Read the model definition and answer for the solid it produces. Units are mm, in the model's axes. A direction names the side the tool comes from. Give positions to 0.01 mm unless a question says otherwise; leave off trailing zeros. Order: outer loops, then holes, each group sorted by start corner. A loop starts at its lowest first (then second) coordinate and runs counter-clockwise, first axis right, second up.
Item 1: The mould has two halves that part along Y. Classify faces 3 (the face through (75, 0, 4)), 4 (the face through (74, 37, 7.873)), 5 (the face through (39.423, 57.426, 6.394)): +Y half, -Y half, draft (parallel to the pull), parting line (faces both ways), or undercut.
Item 2: Which of the six approach directions +Z, -Z, +X, -X, +Y, -Y give full straight-line access (tool end or side, diameter ignored) to faces 1 (the face through (40, 5, 2)), 2 (the face through (136.047, 35.734, 6.394))?
Item 3: A cutting plane is placed at A-A (x = 140). Write down the section's boundary in (y, z).
Item 4: Given pin 1 Ø3 at (x, y) = (15.8, 36.5) entering from -Z; pin 2 Ø3 at (x, y) = (62.5, 35) entering from -Z, each flat-ended and moving along its own axis, determine where each tip first touches the part or whether it passes through.
Item 5: Find the intervals of material crossed by line 1 along X through (y, z) = (11, 1.5); line 2 along Y through (x, z) = (51.25, 5.5); line 3 along X through (y, z) = (13.8, 6.8), in increasing order.
from build123d import *

# Parameters (mm, degrees)
F0_W      = 150
F0_H      = 73
F1_DEPTH  = 7.873
F2_W      = 136
F2_H      = 63
F3_DEPTH  = 4.873
F4_R      = 1.25
F5_DEPTH  = 7.873
F6_R      = 1.25
F7_DEPTH  = 7.873
F8_R      = 1.25
F9_DEPTH  = 7.873
F10_R     = 1.25
F11_DEPTH = 7.873
F12_R     = 1.25
F13_DEPTH = 7.873
F14_R     = 1.25
F15_DEPTH = 7.873
F16_R     = 1.25
F17_DEPTH = 7.873
F18_R     = 1.25
F19_DEPTH = 7.873
F20_R     = 1.25
F21_DEPTH = 7.873
F22_R     = 1.25
F23_DEPTH = 7.873
F24_R     = 1.25
F25_DEPTH = 7.873
F26_R     = 1.25
F27_DEPTH = 7.873
F28_R     = 1.25
F29_DEPTH = 7.873
F30_R     = 1.25
F31_DEPTH = 7.873
F32_R     = 1.25
F33_DEPTH = 7.873
F34_R     = 1.25
F35_DEPTH = 7.873
F36_R     = 1.25
F37_DEPTH = 7.873
F38_R     = 1.25
F39_DEPTH = 7.873
F40_R     = 1.25
F41_DEPTH = 7.873
F42_R     = 1.25
F43_DEPTH = 7.873
F44_R     = 1.25
F45_DEPTH = 7.873
F46_R     = 2
F47_DEPTH = 3
F48_R     = 2
F49_DEPTH = 3
F50_R     = 2
F51_DEPTH = 3
F52_R     = 2
F53_DEPTH = 3
F54_R     = 2
F55_DEPTH = 3
F56_R     = 2
F57_DEPTH = 3
F58_R     = 2
F59_DEPTH = 3
F60_R     = 2
F61_DEPTH = 3
F62_R     = 2
F63_DEPTH = 3
F64_R     = 2
F65_DEPTH = 3
F66_W     = 2.5
F66_H     = 4.873
F67_DEPTH = 63
F68_W     = 2.5
F68_H     = 6.5
F69_DEPTH = 0.623
F70_R     = 2
F71_DEPTH = 3
F73_R     = 2
F74_DEPTH = 3
F75_R     = 2
F76_DEPTH = 3
F77_R     = 2
F78_DEPTH = 3
F79_R     = 2
F80_DEPTH = 3
F72_R     = 2
F81_DEPTH = 3
F82_R     = 1.25
F83_DEPTH = 7.873
F84_R     = 1.25
F85_DEPTH = 7.873


with BuildPart() as f1:
    # F0 (on Top) → F1 (new body)
    with BuildSketch(Plane.XY):
        with Locations((75, 36.5)):
            Rectangle(F0_W, F0_H)
    extrude(amount=F1_DEPTH)

    # F2 (on Top) → F3 (cut)
    with BuildSketch(Plane.XY):
        with Locations((75, 36.5)):
            Rectangle(F2_W, F2_H)
    extrude(amount=F3_DEPTH, mode=Mode.SUBTRACT)

    # F4 (on face) → F5 (cut)
    with BuildSketch(Plane.XY.offset(7.873)):
        with Locations((2.5, 2.5)):
            Circle(F4_R)
    extrude(amount=-F5_DEPTH, mode=Mode.SUBTRACT)

    # F6 (on face) → F7 (cut)
    with BuildSketch(Plane.XY.offset(7.873)):
        with Locations((18, 2.5)):
            Circle(F6_R)
    extrude(amount=-F7_DEPTH, mode=Mode.SUBTRACT)

    # F8 (on face) → F9 (cut)
    with BuildSketch(Plane.XY.offset(7.873)):
        with Locations((34.5, 2.5)):
            Circle(F8_R)
    extrude(amount=-F9_DEPTH, mode=Mode.SUBTRACT)

    # F10 (on face) → F11 (cut)
    with BuildSketch(Plane.XY.offset(7.873)):
        with Locations((51, 2.5)):
            Circle(F10_R)
    extrude(amount=-F11_DEPTH, mode=Mode.SUBTRACT)

    # F12 (on face) → F13 (cut)
    with BuildSketch(Plane.XY.offset(7.873)):
        with Locations((67.5, 2.5)):
            Circle(F12_R)
    extrude(amount=-F13_DEPTH, mode=Mode.SUBTRACT)

    # F14 (on face) → F15 (cut)
    with BuildSketch(Plane.XY.offset(7.873)):
        with Locations((82.5, 2.5)):
            Circle(F14_R)
    extrude(amount=-F15_DEPTH, mode=Mode.SUBTRACT)

    # F16 (on face) → F17 (cut)
    with BuildSketch(Plane.XY.offset(7.873)):
        with Locations((99, 2.5)):
            Circle(F16_R)
    extrude(amount=-F17_DEPTH, mode=Mode.SUBTRACT)

    # F18 (on face) → F19 (cut)
    with BuildSketch(Plane.XY.offset(7.873)):
        with Locations((115.5, 2.5)):
            Circle(F18_R)
    extrude(amount=-F19_DEPTH, mode=Mode.SUBTRACT)

    # F20 (on face) → F21 (cut)
    with BuildSketch(Plane.XY.offset(7.873)):
        with Locations((132, 2.5)):
            Circle(F20_R)
    extrude(amount=-F21_DEPTH, mode=Mode.SUBTRACT)

    # F22 (on face) → F23 (cut)
    with BuildSketch(Plane.XY.offset(7.873)):
        with Locations((147.5, 2.5)):
            Circle(F22_R)
    extrude(amount=-F23_DEPTH, mode=Mode.SUBTRACT)

    # F24 (on face) → F25 (cut)
    with BuildSketch(Plane.XY.offset(7.873)):
        with Locations((2.5, 22)):
            Circle(F24_R)
    extrude(amount=-F25_DEPTH, mode=Mode.SUBTRACT)

    # F26 (on face) → F27 (cut)
    with BuildSketch(Plane.XY.offset(7.873)):
        with Locations((147.5, 22)):
            Circle(F26_R)
    extrude(amount=-F27_DEPTH, mode=Mode.SUBTRACT)

    # F28 (on face) → F29 (cut)
    with BuildSketch(Plane.XY.offset(7.873)):
        with Locations((147.5, 38.5)):
            Circle(F28_R)
    extrude(amount=-F29_DEPTH, mode=Mode.SUBTRACT)

    # F30 (on face) → F31 (cut)
    with BuildSketch(Plane.XY.offset(7.873)):
        with Locations((2.5, 38.5)):
            Circle(F30_R)
    extrude(amount=-F31_DEPTH, mode=Mode.SUBTRACT)

    # F32 (on face) → F33 (cut)
    with BuildSketch(Plane.XY.offset(7.873)):
        with Locations((2.5, 55)):
            Circle(F32_R)
    extrude(amount=-F33_DEPTH, mode=Mode.SUBTRACT)

    # F34 (on face) → F35 (cut)
    with BuildSketch(Plane.XY.offset(7.873)):
        with Locations((147.5, 55)):
            Circle(F34_R)
    extrude(amount=-F35_DEPTH, mode=Mode.SUBTRACT)

    # F36 (on face) → F37 (cut)
    with BuildSketch(Plane.XY.offset(7.873)):
        with Locations((2.5, 70.5)):
            Circle(F36_R)
    extrude(amount=-F37_DEPTH, mode=Mode.SUBTRACT)

    # F38 (on face) → F39 (cut)
    with BuildSketch(Plane.XY.offset(7.873)):
        with Locations((147.5, 70.5)):
            Circle(F38_R)
    extrude(amount=-F39_DEPTH, mode=Mode.SUBTRACT)

    # F40 (on face) → F41 (cut)
    with BuildSketch(Plane.XY.offset(7.873)):
        with Locations((26.25, 70.5)):
            Circle(F40_R)
        Circle(F40_R)
    extrude(amount=-F41_DEPTH, mode=Mode.SUBTRACT)

    # F42 (on face) → F43 (cut)
    with BuildSketch(Plane.XY.offset(7.873)):
        with Locations((123.75, 70.5)):
            Circle(F42_R)
    extrude(amount=-F43_DEPTH, mode=Mode.SUBTRACT)

    # F44 (on face) → F45 (cut)
    with BuildSketch(Plane.XY.offset(7.873)):
        with Locations((75.25, 70.5)):
            Circle(F44_R)
    extrude(amount=-F45_DEPTH, mode=Mode.SUBTRACT)

    # F46 (on face) → F47 (cut)
    with BuildSketch(Plane.XY.offset(7.873)):
        with Locations((38.5, 65.1)):
            Circle(F46_R)
    extrude(amount=-F47_DEPTH, mode=Mode.SUBTRACT)

    # F48 (on face) → F49 (cut)
    with BuildSketch(Plane.XY.offset(7.873)):
        with Locations((38.5, 59.2)):
            Circle(F48_R)
    extrude(amount=-F49_DEPTH, mode=Mode.SUBTRACT)

    # F50 (on face) → F51 (cut)
    with BuildSketch(Plane.XY.offset(7.873)):
        with Locations((15.8, 36.5)):
            Circle(F50_R)
    extrude(amount=-F51_DEPTH, mode=Mode.SUBTRACT)

    # F52 (on face) → F53 (cut)
    with BuildSketch(Plane.XY.offset(7.873)):
        with Locations((67.1, 36.5)):
            Circle(F52_R)
    extrude(amount=-F53_DEPTH, mode=Mode.SUBTRACT)

    # F54 (on face) → F55 (cut)
    with BuildSketch(Plane.XY.offset(7.873)):
        with Locations((111.5, 65.1)):
            Circle(F54_R)
    extrude(amount=-F55_DEPTH, mode=Mode.SUBTRACT)

    # F56 (on face) → F57 (cut)
    with BuildSketch(Plane.XY.offset(7.873)):
        with Locations((111.5, 59.2)):
            Circle(F56_R)
    extrude(amount=-F57_DEPTH, mode=Mode.SUBTRACT)

    # F58 (on face) → F59 (cut)
    with BuildSketch(Plane.XY.offset(7.873)):
        with Locations((82.9, 36.5)):
            Circle(F58_R)
    extrude(amount=-F59_DEPTH, mode=Mode.SUBTRACT)

    # F60 (on face) → F61 (cut)
    with BuildSketch(Plane.XY.offset(7.873)):
        with Locations((134.2, 36.5)):
            Circle(F60_R)
    extrude(amount=-F61_DEPTH, mode=Mode.SUBTRACT)

    # F62 (on face) → F63 (cut)
    with BuildSketch(Plane.XY.offset(7.873)):
        with Locations((58, 19.8)):
            Circle(F62_R)
    extrude(amount=-F63_DEPTH, mode=Mode.SUBTRACT)

    # F64 (on face) → F65 (cut)
    with BuildSketch(Plane.XY.offset(7.873)):
        with Locations((92, 19.8)):
            Circle(F64_R)
    extrude(amount=-F65_DEPTH, mode=Mode.SUBTRACT)

    # F66 (on face) → F67 (join)
    with BuildSketch(Plane(origin=(0, 5, 0), x_dir=(-1, 0, 0), z_dir=(0, 1, 0))):
        with Locations((-75, 2.4365)):
            Rectangle(F66_W, F66_H)
    extrude(amount=F67_DEPTH)

    # F68 (on face) → F69 (cut)
    with BuildSketch(Plane(origin=(0, 0, 0), x_dir=(1, 0, 0), z_dir=(0, 0, -1))):
        with Locations((75, -36.5)):
            Rectangle(F68_W, F68_H)
    extrude(amount=-F69_DEPTH, mode=Mode.SUBTRACT)

    # F70 (on face) → F71 (cut)
    with BuildSketch(Plane(origin=(0, 0, 4.873), x_dir=(1, 0, 0), z_dir=(0, 0, -1))):
        with Locations((38.5, -13.8)):
            Circle(F70_R)
    extrude(amount=-F71_DEPTH, mode=Mode.SUBTRACT)

    # F73 (on face) → F74 (cut)
    with BuildSketch(Plane(origin=(0, 0, 4.873), x_dir=(1, 0, 0), z_dir=(0, 0, -1))):
        with Locations((111.5, -36.5)):
            Circle(F73_R)
    extrude(amount=-F74_DEPTH, mode=Mode.SUBTRACT)

    # F75 (on face) → F76 (cut)
    with BuildSketch(Plane(origin=(0, 0, 4.873), x_dir=(1, 0, 0), z_dir=(0, 0, -1))):
        with Locations((111.5, -13.8)):
            Circle(F75_R)
    extrude(amount=-F76_DEPTH, mode=Mode.SUBTRACT)

    # F77 (on face) → F78 (cut)
    with BuildSketch(Plane(origin=(0, 0, 4.873), x_dir=(1, 0, 0), z_dir=(0, 0, -1))):
        with Locations((61.3, -36.5)):
            Circle(F77_R)
    extrude(amount=-F78_DEPTH, mode=Mode.SUBTRACT)

    # F79 (on face) → F80 (cut)
    with BuildSketch(Plane(origin=(0, 0, 4.873), x_dir=(1, 0, 0), z_dir=(0, 0, -1))):
        with Locations((88.7, -36.5)):
            Circle(F79_R)
    extrude(amount=-F80_DEPTH, mode=Mode.SUBTRACT)

    # F72 (on face) → F81 (cut)
    with BuildSketch(Plane(origin=(0, 0, 4.873), x_dir=(1, 0, 0), z_dir=(0, 0, -1))):
        with Locations((38.5, -36.5)):
            Circle(F72_R)
    extrude(amount=-F81_DEPTH, mode=Mode.SUBTRACT)

    # F82 (on face) → F83 (cut)
    with BuildSketch(Plane(origin=(0, 0, 0), x_dir=(1, 0, 0), z_dir=(0, 0, -1))):
        with Locations((51.25, -70.5)):
            Circle(F82_R)
    extrude(amount=-F83_DEPTH, mode=Mode.SUBTRACT)

    # F84 (on face) → F85 (cut)
    with BuildSketch(Plane(origin=(0, 0, 0), x_dir=(1, 0, 0), z_dir=(0, 0, -1))):
        with Locations((98.75, -70.5)):
            Circle(F84_R)
    extrude(amount=-F85_DEPTH, mode=Mode.SUBTRACT)


solid = f1.part
Response values:
1. face 3: -Y half
1. face 4: draft
1. face 5: undercut
2. face 1: -Z
2. face 2: +Z, -Z
3. outline: (0, 0) - (5, 0) - (5, 4.87) - (68, 4.87) - (68, 0) - (73, 0) - (73, 7.87) - (0, 7.87) - close
4. pin 1: passes through
4. pin 2: stops at z = 4.87
5. line 1: x = 0 to 7, 73.75 to 76.25, 143 to 150
5. line 2: y = 0 to 1.28, 3.72 to 69.25, 71.75 to 73
5. line 3: x = 0 to 36.5, 40.5 to 109.5, 113.5 to 150
